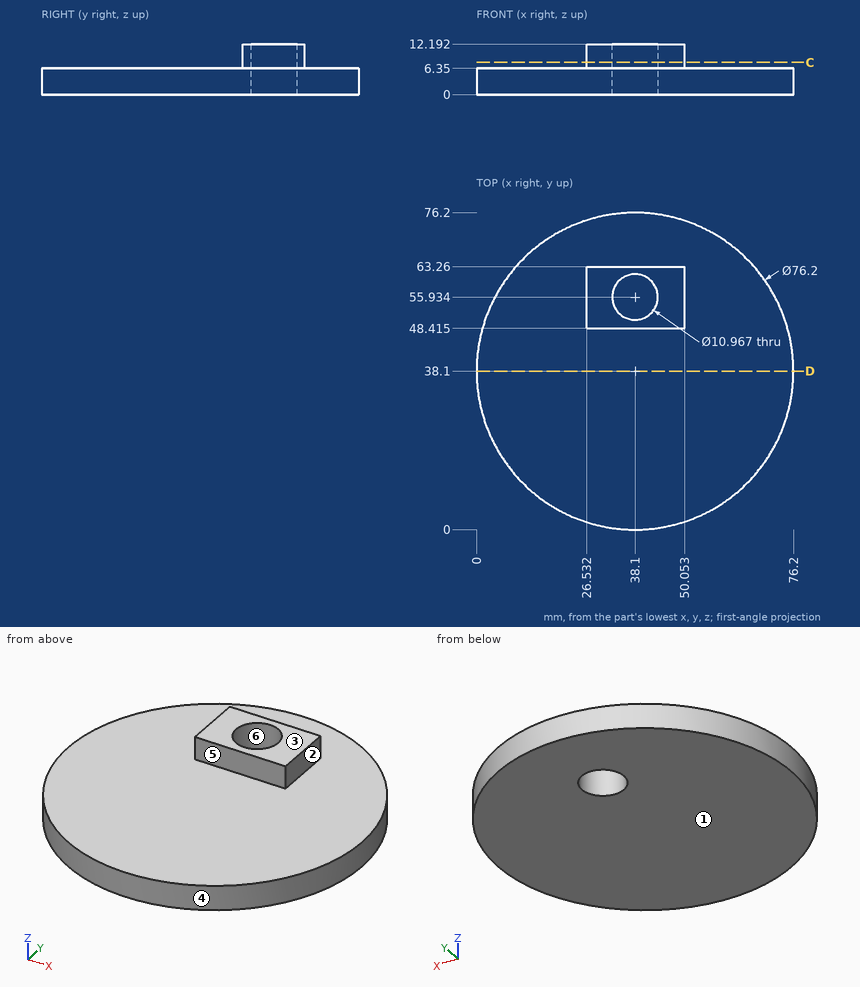
Design review of the part shown in the three views and the two pictorial views. Dimensions are in mm from the part's minimum x, y and z. A direction names the side the tool comes from. Round coordinates to 2 decimals unless told otherwise and drop trailing zeros. Write each loop counter-clockwise with the first axis right and the second up, starting at its lowest first coordinate (ties: lowest second). Pieces come first, ordered by that corner, then holes. Notation, with made-up numbers: M -26,83.25 L 30,83.25 A23 ccw 30,114.25 Z; hole C -18,31.25 d5. An arc over 180 degrees is marked long. Use a Markdown table: item, result. Add a question column.
Q1. The part is to be moulded in two halves that separate along Y. For the marked faces 3, 4, 5 and 6, say which applies: pulls with the +Y half, pulls with the -Y half, needs draft (parallel to the pull), parting line crosses it, or undercut.
Q2. Machinability: for the marked faces 1 and 2, which of the approach directions +Z, -Z, +X, -X, +Y, -Y give a long, thin tool a straight path to every point of the face, cutting with its end or side? Answer none if there is none.
Q3. Insertion check: pin 1 (1.5 mm diameter, centred on y = 14.5, z = 5.5, fed in from -X); pin 2 (1.8 mm diameter, centred on y = 57, z = 10, fed in from +X); pin 3 (3 mm diameter, centred on y = 56.5, z = 10.5, fed in from -X); pin 4 (3 mm diameter, centred on y = 17.5, z = 8.5, fed in from -X). Each pin has a flat end and moves straight along its axis. Give the tip position at first contact, or say it passes through.
Q4. To check wall thickness, follow line 1 (Z direction, x = 58.5, y = 16); line 2 (Y direction, x = 38.1, z = 3.5); line 3 (Y direction, x = 34.5, z = 10) (1 decimal). State the ranges of each line that lie inside material, in increasing order.
Q5. We need section C-C, the plane z = 7.75. State the section outline as (x, y) points (1 decimal), plus the area to 3 significant figures.
Q6. We need section D-D, the plane y = 38.1. State the section outline as (x, z) points.
Findings below:
| question | item | result |
|---|---|---|
| 1 | face 3 | needs draft |
| 1 | face 4 | parting line crosses it |
| 1 | face 5 | pulls with the -Y half |
| 1 | face 6 | undercut |
| 2 | face 1 | -Z, +X, -X, +Y, -Y |
| 2 | face 2 | +Z, +X, +Y, -Y |
| 3 | pin 1 | stops at x = 7.61 |
| 3 | pin 2 | stops at x = 50.05 |
| 3 | pin 3 | stops at x = 26.53 |
| 3 | pin 4 | passes through |
| 4 | line 1 | z = 0 to 6.35 |
| 4 | line 2 | y = 0 to 50.45, 61.42 to 76.2 |
| 4 | line 3 | y = 48.4 to 51.8, 60.1 to 63.3 |
| 5 | outline | M 26.5,48.4 L 50.1,48.4 L 50.1,63.3 L 26.5,63.3 Z; hole C 38.1,55.9 d11 |
| 5 | area | 255 mm² |
| 6 | outline | M 0,0 L 76.2,0 L 76.2,6.35 L 0,6.35 Z |
